Check sheet for the modelled part. Datum: model origin and axes. Units: mm. A direction names the side the tool comes from. Round coordinates to 2 decimals unless told otherwise and drop trailing zeros. Write each loop counter-clockwise with the first axis right and the second up, starting at its lowest first coordinate (ties: lowest second). Pieces come first, ordered by that corner, then holes. Notation, with made-up numbers: (84.25, -17.5) -> (133.25, -17.5) arc R24 cw to (133.25, -4.5) -> close; hole circle Ø4 at (41.25, 81.25). An arc over 180 degrees is marked (long way). Put each result on its own line as item: value. Start each with the question number.
from build123d import *

# Parameters (mm, degrees)
SKETCH1_R           = 7
BOSS_EXTRUDE2_DEPTH = 10
SKETCH3_R           = 56
BOSS_EXTRUDE4_DEPTH = 20
SKETCH5_R           = 3
SKETCH6_R           = 7.5
BOSS_EXTRUDE5_DEPTH = 25
CHAMFER1_SIZE       = 1
SKETCH7_R           = 45
CUT_EXTRUDE2_DEPTH  = 2


with BuildPart() as part:
    # Sketch1 → Boss-Extrude2 (new body)
    with BuildSketch(Plane(origin=(0, 0, 0), x_dir=(1, 0, 0), z_dir=(0, 1, 0))):
        with BuildLine():
            Line((-70.5, 70), (70.5, 70))
            ThreePointArc((70.5, 70), (82.52081528, 65.02081528), (87.5, 53))
            Line((87.5, 53), (87.5, -53))
            ThreePointArc((87.5, -53), (82.52081528, -65.02081528), (70.5, -70))
            Line((70.5, -70), (-70.5, -70))
            ThreePointArc((-70.5, -70), (-82.52081528, -65.02081528), (-87.5, -53))
            Line((-87.5, -53), (-87.5, 53))
            ThreePointArc((-87.5, 53), (-82.52081528, 65.02081528), (-70.5, 70))
        make_face()
        with Locations((-70.5, 53)):
            Circle(SKETCH1_R, mode=Mode.SUBTRACT)
        with Locations((70.5, 53)):
            Circle(SKETCH1_R, mode=Mode.SUBTRACT)
        with Locations((70.5, -53)):
            Circle(SKETCH1_R, mode=Mode.SUBTRACT)
        with Locations((-70.5, -53)):
            Circle(SKETCH1_R, mode=Mode.SUBTRACT)
    extrude(amount=BOSS_EXTRUDE2_DEPTH)

    # Sketch3 → Boss-Extrude4 (add)
    with BuildSketch(Plane(origin=(0, 0, 0), x_dir=(-1, 0, 0), z_dir=(0, -1, 0))):
        Circle(SKETCH3_R)
    extrude(amount=BOSS_EXTRUDE4_DEPTH)

    # Sketch5 → Revolve1 (revolve)
    with BuildSketch(Plane(origin=(0, 0, 0), x_dir=(0, 0, -1), z_dir=(1, 0, 0))):
        with Locations((-56, -17)):
            Circle(SKETCH5_R)
    revolve(axis=Axis((0, 0, 0), (0, -1, 0)))

    # Sketch6 → Boss-Extrude5 (add)
    with BuildSketch(Plane.XZ.offset(20)):
        Circle(SKETCH6_R)
    extrude(amount=BOSS_EXTRUDE5_DEPTH)

    # Chamfer1
    chamfer1_edges = [part.edges().sort_by_distance(p)[0] for p in [
        (-7.5, -45, 0),
    ]]
    chamfer(chamfer1_edges, length=CHAMFER1_SIZE)

    # Sketch7 → Cut-Extrude2 (cut)
    with BuildSketch(Plane(origin=(0, 10, 0), x_dir=(1, 0, 0), z_dir=(0, 1, 0))):
        Circle(SKETCH7_R)
    extrude(amount=-CUT_EXTRUDE2_DEPTH, mode=Mode.SUBTRACT)


solid = part.part
1. Access from +Z, -Z, +X, -X, +Y, -Y to the whole of each face (thin tool, end or side, straight path). Record for faces 4 (the flat face through (-1, 8, -1)), 5 (the cylindrical face through (-51.73, -6.9, 21.45)), 6 (the cylindrical face through (-7.493, -31.832, 0.33)).
2. Material ranges on L1, parallel to Z at x = -70, y = 5; L2, parallel to X at y = 2.25, z = 53; L3, parallel to X at y = 5.5, z = -49, recorded low to high. Write a range as [from, to].
3. Gauge pin test, flat ends, axial feed: P1, Ø16, axis at x = 70.5, z = -53, coming from the -Y side; P2, Ø1, axis at y = -18.5, z = 11, coming from the +X side; P3, Ø1.5, axis at y = -20, z = 5.5, coming from the -X side; P4, Ø22.5, axis at x = -70.5, z = -53, coming from the +Y side. Record the tip position at first contact, or that the pin passes through.
4. Draft check along Z on faces 1 (the cylindrical face through (20.765, 9.014, 39.923)), 2 (the cylindrical face through (82.39, 4.93, -65.15)), 3 (the flat face through (87.5, 5, -1)). Enter one of: released by +Z, released by -Z, zero draft, split by the parting line, or undercut.
5. Section check D-D, the plane y = -38.5. Enter the section's corners in (x, z).
6. Section check B-B, the plane x = 72.5. Enter the section's corners in (y, z).
7. Section check C-C, the plane x = 0. Enter the section's corners in (y, z).
8. Section check A-A, the plane z = 0. Enter the section's corners in (x, y), then the cut area to 3 significant figures.
Reply:
1. face 4: +Y
1. face 5: none
1. face 6: -Y
2. L1: z = [-70, -59.98], [-46.02, 46.02], [59.98, 70]
2. L2: x = [-87.5, -77.5], [-63.5, 63.5], [77.5, 87.5]
2. L3: x = [-87.5, -76.24], [-64.76, 64.76], [76.24, 87.5]
3. P1: stops at y = 0
3. P2: stops at x = 57.81
3. P3: stops at x = -57.73
3. P4: stops at y = 10
4. face 1: undercut
4. face 2: released by -Z
4. face 3: zero draft
5. outline: circle Ø15 at (0, 0)
6. outline: (0, -69.88) -> (10, -69.88) -> (10, -59.71) -> (0, -59.71) -> close; (0, -46.29) -> (10, -46.29) -> (10, 46.29) -> (0, 46.29) -> close; (0, 59.71) -> (10, 59.71) -> (10, 69.88) -> (0, 69.88) -> close
7. outline: (-45, -6.5) -> (-44, -7.5) -> (-20, -7.5) -> (-20, -56) arc R3 ccw to (-14, -56) -> (0, -56) -> (0, -70) -> (10, -70) -> (10, -45) -> (8, -45) -> (8, 45) -> (10, 45) -> (10, 70) -> (0, 70) -> (0, 56) -> (-14, 56) arc R3 ccw to (-20, 56) -> (-20, 7.5) -> (-44, 7.5) -> (-45, 6.5) -> close
8. outline: (-87.5, 0) -> (-56, 0) -> (-56, -14) arc R3 ccw to (-56, -20) -> (-7.5, -20) -> (-7.5, -44) -> (-6.5, -45) -> (6.5, -45) -> (7.5, -44) -> (7.5, -20) -> (56, -20) arc R3 ccw to (56, -14) -> (56, 0) -> (87.5, 0) -> (87.5, 10) -> (45, 10) -> (45, 8) -> (-45, 8) -> (-45, 10) -> (-87.5, 10) -> close
8. area: 4,210 mm2
